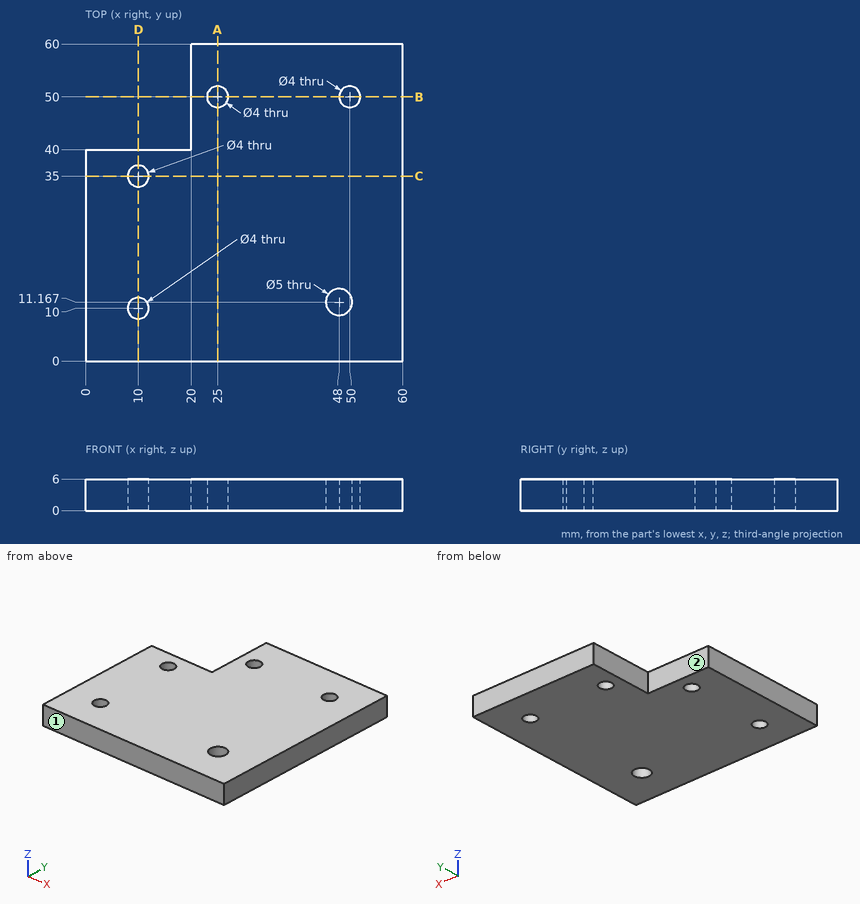
Could you check a few things on this drawing? It's one solid part, dimensions in mm from its lowest x, y, z. A direction names the side the tool comes from. Coordinates: 2 decimals unless noted, no trailing zeros. Order: outer loops, then holes, each group sorted by start corner. A loop starts at its lowest first (then second) coordinate and runs counter-clockwise, first axis right, second up.
1. For the marked faces 1 and 2, which set-ups out of +Z, -Z, +X, -X, +Y, -Y let a thin tool reach every point of the face, with its end or its side?
2. If we section it at C-C (y = 35): Please give me the cut outline in (x, z), then the cut area to 3 significant figures.
3. I need wall thicknesses on line 1 (Y direction, x = 9.5, z = 1.9); line 2 (Y direction, x = 10, z = 2.1); line 3 (Y direction, x = 25, z = 1.35). Which ranges of each line are inside material? Lowest first, please.
4. If we section it at D-D (x = 10): Please give me the cut outline in (y, z), then the cut area to 3 significant figures.
5. If we section it at B-B (y = 50): Please give me the cut outline in (x, z), then the cut area to 3 significant figures.
6. If we section it at A-A (x = 25): Please give me the cut outline in (y, z), then the cut area to 3 significant figures.
Entries:
1. face 1: +Z, -Z, +X, -X, -Y
1. face 2: +Z, -Z, -X, +Y
2. outline: (0, 0) - (8, 0) - (8, 6) - (0, 6) - close; (12, 0) - (60, 0) - (60, 6) - (12, 6) - close
2. area: 336 mm2
3. line 1: y = 0 to 8.06, 11.94 to 33.06, 36.94 to 40
3. line 2: y = 0 to 8, 12 to 33, 37 to 40
3. line 3: y = 0 to 48, 52 to 60
4. outline: (0, 0) - (8, 0) - (8, 6) - (0, 6) - close; (12, 0) - (33, 0) - (33, 6) - (12, 6) - close; (37, 0) - (40, 0) - (40, 6) - (37, 6) - close
4. area: 192 mm2
5. outline: (20, 0) - (23, 0) - (23, 6) - (20, 6) - close; (27, 0) - (48, 0) - (48, 6) - (27, 6) - close; (52, 0) - (60, 0) - (60, 6) - (52, 6) - close
5. area: 192 mm2
6. outline: (0, 0) - (48, 0) - (48, 6) - (0, 6) - close; (52, 0) - (60, 0) - (60, 6) - (52, 6) - close
6. area: 336 mm2
